The model under review builds one solid part; all positions refer to its coordinate system, in mm. A direction names the side the tool comes from. Coordinates: 2 decimals unless noted, no trailing zeros. Write each loop counter-clockwise with the first axis right and the second up, starting at its lowest first coordinate (ties: lowest second). Pieces come first, ordered by that corner, then holes. Notation, with made-up numbers: (-2.75, -15) -> (44.25, -15) arc R17 ccw to (44.25, 1) -> close; hole circle Ø4 at (-27, 29). An arc over 180 degrees is marked (long way). Write each question's results on one line, items separated by ' | '.
```python
from build123d import *

# Parameters (mm, degrees)
BOSS_EXTRUDE1_DEPTH = 45
BOSS_EXTRUDE2_DEPTH = 3
FILLET1_R           = 2
SKETCH5_R           = 1.4
CUT_EXTRUDE1_DEPTH  = 68.3348504


with BuildPart() as part:
    # Sketch3 → Boss-Extrude1 (new body)
    with BuildSketch(Plane(origin=(0, 0, 0), x_dir=(1, 0, 0), z_dir=(0, 1, 0))):
        with BuildLine():
            Line((-8, 24), (-22.053839059, 24))
            ThreePointArc((-22.053839059, 24), (-22.90912017, 23.807897735), (-23.600099843, 23.268494221))
            Line((-23.600099843, 23.268494221), (-37.546260784, 6.268494221))
            ThreePointArc((-37.546260784, 6.268494221), (-37.883151822, 5.673601675), (-38, 5))
            Line((-38, 5), (-38, -5))
            ThreePointArc((-38, -5), (-37.883151822, -5.673601675), (-37.546260784, -6.268494221))
            Line((-37.546260784, -6.268494221), (-23.600099843, -23.268494221))
            ThreePointArc((-23.600099843, -23.268494221), (-22.90912017, -23.807897735), (-22.053839059, -24))
            Line((-22.053839059, -24), (-8, -24))
            Line((-8, -24), (-8, -27))
            Line((-8, -27), (-22.053839059, -27))
            ThreePointArc((-22.053839059, -27), (-24.192041837, -26.519744338), (-25.919491019, -25.171235552))
            Line((-25.919491019, -25.171235552), (-39.86565196, -8.171235552))
            ThreePointArc((-39.86565196, -8.171235552), (-40.707879555, -6.684004186), (-41, -5))
            Line((-41, -5), (-41, 5))
            ThreePointArc((-41, 5), (-40.707879555, 6.684004186), (-39.86565196, 8.171235552))
            Line((-39.86565196, 8.171235552), (-25.919491019, 25.171235552))
            ThreePointArc((-25.919491019, 25.171235552), (-24.192041837, 26.519744338), (-22.053839059, 27))
            Line((-22.053839059, 27), (-8, 27))
            Line((-8, 27), (-8, 24))
        make_face()
    extrude(amount=BOSS_EXTRUDE1_DEPTH)

    # Sketch4 → Boss-Extrude2 (add)
    with BuildSketch(Plane.XZ.offset(-45)):
        Polygon((-28.135718162, 22.469713492), (-35.867022082, 28.812184595), (-45.380728737, 17.215228715), (-37.649424817, 10.872757612), align=None)
        Polygon((-37.649424817, -10.872757612), (-45.380728737, -17.215228715), (-35.867022082, -28.812184595), (-28.135718162, -22.469713492), align=None)
    extrude(amount=BOSS_EXTRUDE2_DEPTH)

    # Fillet1
    fillet1_edges = [part.edges().sort_by_distance(p)[0] for p in [
        (-35.867022082, 43.5, 28.812184595),
        (-45.380728737, 43.5, 17.215228715),
        (-32.892571489, 42, 16.671235552),
        (-45.380728737, 43.5, -17.215228715),
        (-35.867022082, 43.5, -28.812184595),
        (-32.892571489, 42, -16.671235552),
    ]]
    fillet(fillet1_edges, radius=FILLET1_R)

    # Sketch5 → Cut-Extrude1 (cut, through all)
    with BuildSketch(Plane.XZ.offset(-42)):
        with Locations(Location((-37.531353842, 20.476718214, 0), (0, 0, 270))):
            Circle(SKETCH5_R)
    cut_extrude1 = extrude(amount=-CUT_EXTRUDE1_DEPTH, mode=Mode.SUBTRACT)

    # Mirror1: Cut-Extrude1 across plane
    add(cut_extrude1.mirror(Plane.XY), mode=Mode.SUBTRACT)


solid = part.part
```
Q1. Machinability: for faces 5 (the cylindrical face through (-35.76, 43.48, -27.99)), 6 (the flat face through (-37, 42, 22)), 7 (the flat face through (-15, 22, -24)), which of the approach directions +Z, -Z, +X, -X, +Y, -Y give a long, thin tool a straight path to every point of the face, cutting with its end or side? Answer none if there is none.
Solution:
face 5: -Z, +Y, -Y | face 6: +Z, -X, -Y | face 7: +X, +Y, -Y
Q2. Add section B-B (y = 34.5). Write out the cut boundary in (x, z).
Solution:
outline: (-41, -5) arc R5 ccw to (-39.87, -8.17) -> (-25.92, -25.17) arc R5 ccw to (-22.05, -27) -> (-8, -27) -> (-8, -24) -> (-22.05, -24) arc R2 cw to (-23.6, -23.27) -> (-37.55, -6.27) arc R2 cw to (-38, -5) -> (-38, 5) arc R2 cw to (-37.55, 6.27) -> (-23.6, 23.27) arc R2 cw to (-22.05, 24) -> (-8, 24) -> (-8, 27) -> (-22.05, 27) arc R5 ccw to (-25.92, 25.17) -> (-39.87, 8.17) arc R5 ccw to (-41, 5) -> close
Q3. Add section C-C (z = 2). Write out the cut boundary in (x, y).
Solution:
outline: (-41, 0) -> (-38, 0) -> (-38, 45) -> (-41, 45) -> close
Q4. Add section A-A (x = -13.5). Write out the cut boundary in (y, z), plus the area to 3 significant figures.
Solution:
outline: (0, -27) -> (45, -27) -> (45, -24) -> (0, -24) -> close; (0, 24) -> (45, 24) -> (45, 27) -> (0, 27) -> close | area: 270 mm²
Q5. Draft analysis for pull direction Z (two halves, no side actions). For faces 1 (the cylindrical face through (-24.22, 22.185, -26.506)), 2 (the cylindrical face through (-35.76, 43.48, 27.99)), 3 (the flat face through (-38.4, 45, -0.1)), 4 (the flat face through (-15, 22, 24)), state which applies: pulls with the +Z half, pulls with the -Z half, needs draft (parallel to the pull), parting line crosses it, or undercut.
Solution:
face 1: pulls with the -Z half | face 2: pulls with the +Z half | face 3: needs draft | face 4: undercut
Q6. Add section D-D (x = -24.5). Write out the cut boundary in (y, z), plus the area to 3 significant figures.
Solution:
outline: (0, -26.36) -> (45, -26.36) -> (45, -22.17) -> (0, -22.17) -> close; (0, 22.17) -> (45, 22.17) -> (45, 26.36) -> (0, 26.36) -> close | area: 377 mm²
Q7. For line 1 (Z direction, x = -20, y = 40); line 2 (Z direction, x = -28, y = 4); line 3 (X direction, y = 42, z = 3), list the stretches that pass through material, from the lowest coordinate up. Write a range as from..to.
Solution:
line 1: -27..-24, 24..27 | line 2: -22.64..-17.91, 17.91..22.64 | line 3: -41..-38
Q8. Clearance check with flat-ended pins moving along their axes: P1, Ø12, axis at x = -37, z = 23.5, coming from the -Y side; P2, Ø1, axis at x = -36, y = 8.5, coming from the +Z side; P3, Ø1.5, axis at x = -12, y = 26, coming from the -Z side. State where each tip first meets the part, or that it passes through.
Solution:
P1: y = 41.94 | P2: z = 13.49 | P3: z = -27
